```python
from build123d import *

# Parameters (mm, degrees)
ESQUISSE1_W             = 85
ESQUISSE1_H             = 85
BOSS_EXTRU_1_DEPTH      = 105
ESQUISSE2_W             = 25
ESQUISSE2_H             = 20
BOSS_EXTRU_2_DEPTH      = 105
ESQUISSE3_R             = 5
ENL_V_MAT_EXTRU_1_DEPTH = 106
BOSS_EXTRU_3_REACH      = 107
ESQUISSE5_W             = 25
ESQUISSE5_H             = 7.5
CONG_1_R                = 10
ESQUISSE6_W             = 40
ESQUISSE6_H             = 40
ESQUISSE6_W_2           = 20
ESQUISSE6_H_2           = 20.000133682
BOSS_EXTRU_5_DEPTH      = 83
BOSS_EXTRU_5_DEPTH_BACK = 176
ESQUISSE7_W             = 67.482972399
ESQUISSE7_H             = 90.273524416
ESQUISSE7_H_2           = 40
ENL_V_MAT_EXTRU_2_DEPTH = 106
ESQUISSE8_W             = 40
ESQUISSE8_H             = 25.5
ENL_V_MAT_EXTRU_3_DEPTH = 73.5
ESQUISSE9_W             = 20
ESQUISSE9_H             = 20
BOSS_EXTRU_7_DEPTH      = 40
ESQUISSE11_W            = 40.341877054
ESQUISSE11_H            = 20
BOSS_EXTRU_8_DEPTH      = 32.5
ESQUISSE12_W            = 40
ESQUISSE12_H            = 20
BOSS_EXTRU_9_DEPTH      = 32.5
ESQUISSE13_R            = 5
ENL_V_MAT_EXTRU_4_DEPTH = 106
BOSS_EXTRU_11_DEPTH     = 105
BOSS_EXTRU_12_REACH     = 152.5
ESQUISSE15_W            = 107.018090517
ESQUISSE15_H            = 7.5
CONG_2_R                = 10
CONG_3_R                = 10
ENL_V_MAT_EXTRU_6_DEPTH = 57.25
CONG_4_R                = 10
ENL_V_MAT_EXTRU_7_DEPTH = 151.5
ENL_V_MAT_EXTRU_8_DEPTH = 151.5
ENL_V_MAT_EXTRU_9_DEPTH = 151.5


with BuildPart() as part:
    # Esquisse1 → Boss.-Extru.1 (new body)
    with BuildSketch(Plane.XY):
        Polygon((-48.567045776, 45.091911765), (-95.067045776, 52.5), (-153.567045776, 52.5), (-153.567045776, -52.5), (-95.067045776, -52.5), (-48.567045776, -45.091911765), align=None)
        with Locations((-101.067045776, 0)):
            Rectangle(ESQUISSE1_W, ESQUISSE1_H, mode=Mode.SUBTRACT)
    extrude(amount=BOSS_EXTRU_1_DEPTH)

    # Esquisse2 → Boss.-Extru.2 (add, through all)
    with BuildSketch(Plane.XZ.offset(52.5)):
        with Locations((-36.067045776, 10)):
            Rectangle(ESQUISSE2_W, ESQUISSE2_H)
    extrude(amount=-BOSS_EXTRU_2_DEPTH)

    # Esquisse3 → Enlèv. mat.-Extru.1 (cut, through all)
    with BuildSketch(Plane.XZ.offset(52.5)):
        with Locations((-33.567045776, 10)):
            Circle(ESQUISSE3_R)
    extrude(amount=-ENL_V_MAT_EXTRU_1_DEPTH, mode=Mode.SUBTRACT)

    # Esquisse5 → Boss.-Extru.3 (add, up to next)
    with BuildSketch(Plane.XY.offset(105), mode=Mode.PRIVATE) as boss_extru_3_sk1:
        with Locations((-36.067045776, 0)):
            Rectangle(ESQUISSE5_W, ESQUISSE5_H)
    boss_extru_3_tool1 = extrude(boss_extru_3_sk1.sketch, amount=-BOSS_EXTRU_3_REACH, mode=Mode.PRIVATE) - part.part
    add(boss_extru_3_tool1.solids().sort_by_distance((-36.067046, 0, 105))[0])

    # Congé1
    cong_1_edges = [part.edges().sort_by_distance(p)[0] for p in [
        (-23.567045776, 28.125, 20),
        (-23.567045776, -28.125, 20),
    ]]
    fillet(cong_1_edges, radius=CONG_1_R)



with BuildPart() as body_2:
    # Esquisse6 → Boss.-Extru.5 (new body, two sides)
    with BuildSketch(Plane(origin=(0, 0, 0), x_dir=(-1, 0, 0), z_dir=(0, 0, -1))) as boss_extru_5_sk:
        with Locations((-103.451044741, 0)):
            Rectangle(ESQUISSE6_W, ESQUISSE6_H)
        with Locations((-103.451044741, 0)):
            Rectangle(ESQUISSE6_W_2, ESQUISSE6_H_2, mode=Mode.SUBTRACT)
    extrude(amount=BOSS_EXTRU_5_DEPTH)
    extrude(boss_extru_5_sk.sketch, amount=-BOSS_EXTRU_5_DEPTH_BACK)

    # Esquisse7 → Enlèv. mat.-Extru.2 (cut, through all)
    with BuildSketch(Plane.XZ.offset(52.5)):
        with Locations((109.464150934, -45.136762208)):
            Rectangle(ESQUISSE7_W, ESQUISSE7_H)
        with Locations((109.464150934, 20)):
            Rectangle(ESQUISSE7_W, ESQUISSE7_H_2)
    extrude(amount=-ENL_V_MAT_EXTRU_2_DEPTH, mode=Mode.SUBTRACT)

    # Esquisse8 → Enlèv. mat.-Extru.3 (cut, through all)
    with BuildSketch(Plane.XZ.offset(20)):
        with Locations((103.451044741, 163.25)):
            Rectangle(ESQUISSE8_W, ESQUISSE8_H)
    extrude(amount=-ENL_V_MAT_EXTRU_3_DEPTH, mode=Mode.SUBTRACT)

    # Esquisse9 → Boss.-Extru.7 (add)
    with BuildSketch(Plane(origin=(0, -20, 0), x_dir=(-1, 0, 0), z_dir=(0, -1, 0))):
        with Locations((-73.451044741, -50)):
            Rectangle(ESQUISSE9_W, ESQUISSE9_H)
    extrude(amount=-BOSS_EXTRU_7_DEPTH)

    # Esquisse11 → Boss.-Extru.8 (add)
    with BuildSketch(Plane.XZ.offset(52.5)):
        with Locations((83.621983268, 50)):
            Rectangle(ESQUISSE11_W, ESQUISSE11_H)
    extrude(amount=-BOSS_EXTRU_8_DEPTH)

    # Esquisse12 → Boss.-Extru.9 (add)
    with BuildSketch(Plane(origin=(0, 52.5, 0), x_dir=(1, 0, 0), z_dir=(0, 1, 0))):
        with Locations((83.451044741, -50)):
            Rectangle(ESQUISSE12_W, ESQUISSE12_H)
    extrude(amount=-BOSS_EXTRU_9_DEPTH)

    # Esquisse13 → Enlèv. mat.-Extru.4 (cut, through all)
    with BuildSketch(Plane.XZ.offset(52.5)):
        with Locations((73.451044741, 50)):
            Circle(ESQUISSE13_R)
    extrude(amount=-ENL_V_MAT_EXTRU_4_DEPTH, mode=Mode.SUBTRACT)


with BuildPart() as part_1:
    add(part.part)

    add(body_2.part)  # Boss.-Extru.11 merges body 2
    # Esquisse14 → Boss.-Extru.11 (add, through all)
    with BuildSketch(Plane.XZ.offset(52.5)):
        with BuildLine():
            Line((-23.567045776, 0), (-1.074115191, 0))
            ThreePointArc((-1.074115191, 0), (3.110427636, 0.917621383), (6.527005267, 3.502079733))
            Line((6.527005267, 3.502079733), (34.733944249, 36.497920267))
            ThreePointArc((34.733944249, 36.497920267), (38.15052188, 39.082378617), (42.335064706, 40))
            Line((42.335064706, 40), (63.451044741, 40))
            Line((63.451044741, 40), (63.451044741, 46))
            Line((63.451044741, 46), (42.335064706, 46))
            ThreePointArc((42.335064706, 46), (38.15052188, 45.082378617), (34.733944249, 42.497920267))
            Line((34.733944249, 42.497920267), (6.527005267, 9.502079733))
            ThreePointArc((6.527005267, 9.502079733), (3.110427636, 6.917621383), (-1.074115191, 6))
            Line((-1.074115191, 6), (-23.567045776, 6))
            Line((-23.567045776, 6), (-23.567045776, 0))
        make_face()
    extrude(amount=-BOSS_EXTRU_11_DEPTH)

    # Esquisse15 → Boss.-Extru.12 (add, up to next)
    with BuildSketch(Plane.XY.offset(150.5), mode=Mode.PRIVATE) as boss_extru_12_sk1:
        with Locations((29.941999483, 0)):
            Rectangle(ESQUISSE15_W, ESQUISSE15_H)
    boss_extru_12_tool1 = extrude(boss_extru_12_sk1.sketch, amount=-BOSS_EXTRU_12_REACH, mode=Mode.PRIVATE) - part_1.part
    add(boss_extru_12_tool1.solids().sort_by_distance((29.941999, 0, 150.5))[0])

    # Congé2
    cong_2_edges = [part_1.edges().sort_by_distance(p)[0] for p in [
        (63.451044741, -28.125, 60),
    ]]
    fillet(cong_2_edges, radius=CONG_2_R)

    # Congé3
    cong_3_edges = [part_1.edges().sort_by_distance(p)[0] for p in [
        (63.451044741, 28.125, 60),
    ]]
    fillet(cong_3_edges, radius=CONG_3_R)

    # Esquisse16 → Enlèv. mat.-Extru.6 (cut, through all)
    with BuildSketch(Plane.XZ.offset(3.75)):
        with BuildLine():
            Line((60.598915971, 150.5), (26.069543092, 108.637003713))
            ThreePointArc((26.069543092, 108.637003713), (22.619512531, 105.954836572), (18.355122942, 105))
            Line((18.355122942, 105), (-23.567045776, 105))
            Line((-23.567045776, 105), (-23.567045776, 150.5))
            Line((-23.567045776, 150.5), (60.598915971, 150.5))
        make_face()
    extrude(amount=-ENL_V_MAT_EXTRU_6_DEPTH, mode=Mode.SUBTRACT)

    # Congé4
    cong_4_edges = [part_1.edges().sort_by_distance(p)[0] for p in [
        (60.598915971, 0, 150.5),
    ]]
    fillet(cong_4_edges, radius=CONG_4_R)

    # Esquisse17 → Enlèv. mat.-Extru.7 (cut, through all)
    with BuildSketch(Plane.XY.offset(150.5)):
        Polygon((-93.466358172, -52.244988494), (103.792921795, -20), (103.792921795, -55.275638449), align=None)
    extrude(amount=-ENL_V_MAT_EXTRU_7_DEPTH, mode=Mode.SUBTRACT)

    # Esquisse18 → Enlèv. mat.-Extru.8 (cut, through all)
    with BuildSketch(Plane.XY.offset(150.5)):
        Polygon((-92.222865715, 52.046883079), (103.451044741, 20), (103.451044741, 52.5), align=None)
    extrude(amount=-ENL_V_MAT_EXTRU_8_DEPTH, mode=Mode.SUBTRACT)

    # Esquisse19 → Enlèv. mat.-Extru.9 (cut, through all)
    with BuildSketch(Plane.XY.offset(150.5)):
        Polygon((-79.463248921, 79.178617238), (139.979375794, 56.935567532), (111.241114329, 33.487041007), (-48.920553802, 47.63996467), align=None)
    extrude(amount=-ENL_V_MAT_EXTRU_9_DEPTH, mode=Mode.SUBTRACT)


solid = part_1.part
```
The listing builds one solid part. Answer for the finished solid, in the listing's coordinates (mm). A direction names the side the tool comes from. Coordinates: 2 decimals unless noted, no trailing zeros. Loops run counter-clockwise (first coordinate to the right, second up) from the corner with the lowest first, then second, coordinate; pieces in that order, holes last. Notation, with made-up numbers: (39.5, 87.5) - (71.5, 87.5) arc R17 cw to (71.5, 102.5) - close; hole circle Ø2 at (4, -21.75). An arc over 180 degrees is marked (long way). Use a Markdown table: item, result. Add a question column.
1) For faces 4 (the cylindrical face through (-26.574, -22.831, 17.148)), 5 (the flat face through (73, 0, 40)), 6 (the flat face through (-55, 0, 105)), 7 (the cylindrical face through (66.46, 15.31, 57.15)), 8 (the flat face through (-143.567, -1, 52)), determine the directions among +Z, -Z, +X, -X, +Y, -Y from which every point of the face is accessible in a straight line to the end or side of a thin tool.
2) The mould has two halves that part along X. Classify faces 1 (the flat face through (-52.82, 45.594, 48.856)), 2 (the flat face through (104, 20, 94)), 3 (the flat face through (104, -10, 94)): released by +X, released by -X, zero draft, split by the parting line, or undercut.
3) The part is cut by section D-D, the plane z = 128. Give the vertices of the cut face in (x, y).
4) The part is cut by section A-A, the plane y = 15.5. Give the vertices of the cut face in (x, z), and give its area (3 significant figures).
5) The part is cut by section C-C, the plane x = -75. Give the vertices of the cut face in (y, z), and give its area (3 significant figures).
6) Find the intervals of material crossed by line 1 (X direction, y = -14.5, z = 50); line 2 (X direction, y = 3, z = 50); line 3 (X direction, y = -5, z = 50), in increasing order.
7) Given pin 1 (2 mm diameter, centred on y = -16, z = 8.5, fed in from +X); pin 2 (6.5 mm diameter, centred on x = 51.5, y = -10.5, fed in from +Z); pin 3 (1 mm diameter, centred on x = 6, z = 98.5, fed in from -Y), each flat-ended and moving along its own axis, determine where each tip first touches the part or whether it passes through.
8) The part is cut by section B-B, the plane z = 76. Give the vertices of the cut face in (x, y), and give its area (3 significant figures).
Here are the results:
| question | item | result |
|---|---|---|
| 1 | face 4 | +Z, -Y |
| 1 | face 5 | -Z, +X, +Y, -Y |
| 1 | face 6 | +Z, -X, +Y, -Y |
| 1 | face 7 | +Z, +Y |
| 1 | face 8 | +Z, -Z |
| 2 | face 1 | released by +X |
| 2 | face 2 | zero draft |
| 2 | face 3 | undercut |
| 3 | outline | (42.04, -3.75) - (83.45, -3.75) - (83.45, -20) - (123.45, -20) - (123.45, 20) - (83.45, 20) - (83.45, 3.75) - (42.04, 3.75) - close; hole (93.45, -10) - (113.45, -10) - (113.45, 10) - (93.45, 10) - close |
| 4 | outline | (-153.57, 0) - (-143.57, 0) - (-143.57, 105) - (-153.57, 105) - close; (-58.57, 0) - (-1.07, 0) arc R10 ccw to (6.53, 3.5) - (34.73, 36.5) arc R10 cw to (42.34, 40) - (123.45, 40) - (123.45, 150.5) - (83.45, 150.5) - (83.45, 60) - (73.45, 60) arc R10 ccw to (63.45, 50) - (63.45, 46) - (42.34, 46) arc R10 ccw to (34.73, 42.5) - (6.53, 9.5) arc R10 cw to (-1.07, 6) - (-23.57, 6) - (-23.57, 10) arc R10 ccw to (-33.57, 20) - (-48.57, 20) - (-48.57, 105) - (-58.57, 105) - close; hole circle Ø10 at (-33.57, 10); hole circle Ø10 at (73.45, 50) |
| 4 | area | 7,740 mm^2 |
| 5 | outline | (-49.23, 0) - (-42.5, 0) - (-42.5, 105) - (-49.23, 105) - close; (42.5, 0) - (49.23, 0) - (49.23, 105) - (42.5, 105) - close |
| 5 | area | 1,410 mm^2 |
| 6 | line 1 | x = -153.57 to -143.57, -58.57 to -48.57, 63.45 to 68.45, 78.45 to 123.45 |
| 6 | line 2 | x = -153.57 to -143.57, -58.57 to 68.45, 78.45 to 93.45, 113.45 to 123.45 |
| 6 | line 3 | x = -153.57 to -143.57, -58.57 to -48.57, 63.45 to 68.45, 78.45 to 93.45, 113.45 to 123.45 |
| 7 | pin 1 | stops at x = 11.65 |
| 7 | pin 2 | stops at z = 46 |
| 7 | pin 3 | stops at y = -3.75 |
| 8 | outline | (-153.57, -52.5) - (-95.07, -52.5) - (-93.47, -52.24) - (-48.57, -44.91) - (-48.57, -3.75) - (83.45, -3.75) - (83.45, -20) - (123.45, -20) - (123.45, 20) - (83.45, 20) - (83.45, 3.75) - (-48.57, 3.75) - (-48.57, 44.9) - (-92.22, 52.05) - (-95.07, 52.5) - (-153.57, 52.5) - close; hole (-143.57, -42.5) - (-58.57, -42.5) - (-58.57, 42.5) - (-143.57, 42.5) - close; hole (93.45, -10) - (113.45, -10) - (113.45, 10) - (93.45, 10) - close |
| 8 | area | 5,640 mm^2 |
